from build123d import *

# Parameters (mm, degrees)
SKETCH1_R           = 3.175
BOSS_EXTRUDE1_DEPTH = 6.35


with BuildPart() as part:
    # Sketch1 → Boss-Extrude1 (new body)
    with BuildSketch(Plane.XY):
        Polygon((38.1, 12.7), (114.3, 12.7), (114.3, 17.050166685), (139.7, 17.050166685), (139.7, 12.7), (152.4, 12.7), (152.4, 0), (0, 0), (0, 12.7), (12.7, 12.7), (12.7, 17.050166685), (38.1, 17.050166685), align=None)
        with Locations((50.8, 6.35)):
            Circle(SKETCH1_R, mode=Mode.SUBTRACT)
        with Locations((76.2, 6.35)):
            Circle(SKETCH1_R, mode=Mode.SUBTRACT)
        with Locations((101.6, 6.35)):
            Circle(SKETCH1_R, mode=Mode.SUBTRACT)
    extrude(amount=BOSS_EXTRUDE1_DEPTH)


solid = part.part
Input: part model. Units: mm. Frame: model coordinates. A direction names the side the tool comes from. Coordinates: 2 decimals unless noted, no trailing zeros. Loops run counter-clockwise (first coordinate to the right, second up) from the corner with the lowest first, then second, coordinate; pieces in that order, holes last. Notation, with made-up numbers: (12, -30.75) -> (71, -30.75) arc R25 ccw to (71, -8.75) -> close; hole circle Ø3 at (-24.75, 29). An arc over 180 degrees is marked (long way). Write each question's results on one line, items separated by ' | '. Start each with the question number.
Q1. Pull-direction query (Y, two-part tool) for faces 6 (the flat face through (127, 17.05, 3)), 7 (the cylindrical face through (98.43, 6.49, 3.13)), 8 (the cylindrical face through (53.83, 7.3, 3.13)), 9 (the flat face through (77, 11, 6.35)); classes: released by +Y, released by -Y, zero draft, split by the parting line, or undercut.
Q2. Section B-B, the plane x = 50.8. Return the cut outline in (y, z) (3 decimals), plus the area to 3 significant figures.
Q3. Ray query, line 1 (X direction, y = 6.25, z = 3.5); line 2 (X direction, y = 9, z = 4); line 3 (Y direction, x = 76.2, z = 3) (3 decimals). Return the intervals inside material, ascending. Write a range as from..to.
Q4. Section C-C, the plane z = 1. Return the cut outline in (x, y) (3 decimals).
Q5. Reachability of faces 1 (the flat face through (6, 12.7, 3)), 2 (the flat face through (25, 17.05, 3)), 3 (the flat face through (146, 12.7, 3)), 4 (the flat face through (114.3, 15, 3)), 5 (the flat face through (77, 11, 0)) from +Z, -Z, +X, -X, +Y, -Y: full face, straight path, thin tool, end or side. Return the list, or none.
Q6. Pin query (flat end, axial travel): pin 1 (2 mm diameter, centred on y = 16, z = 3, fed in from +X); pin 2 (3 mm diameter, centred on x = 85.5, z = 3.5, fed in from +Y); pin 3 (1 mm diameter, centred on x = 98, y = 15, fed in from +Z). Return the tip coordinate at first contact, or that it passes through.
Q7. Section A-A, the plane y = 6.35. Return the cut outline in (x, z) (3 decimals).
Found:
1) face 6: released by +Y | face 7: undercut | face 8: undercut | face 9: zero draft
2) outline: (0, 0) -> (3.175, 0) -> (3.175, 6.35) -> (0, 6.35) -> close; (9.525, 0) -> (12.7, 0) -> (12.7, 6.35) -> (9.525, 6.35) -> close | area: 40.3 mm2
3) line 1: 0..47.63, 53.97..73.03, 79.37..98.43, 104.77..152.4 | line 2: 0..49.05, 52.55..74.45, 77.95..99.85, 103.35..152.4 | line 3: 0..3.175, 9.525..12.7
4) outline: (0, 0) -> (152.4, 0) -> (152.4, 12.7) -> (139.7, 12.7) -> (139.7, 17.05) -> (114.3, 17.05) -> (114.3, 12.7) -> (38.1, 12.7) -> (38.1, 17.05) -> (12.7, 17.05) -> (12.7, 12.7) -> (0, 12.7) -> close; hole circle Ø6.35 at (50.8, 6.35); hole circle Ø6.35 at (76.2, 6.35); hole circle Ø6.35 at (101.6, 6.35)
5) face 1: +Z, -Z, -X, +Y | face 2: +Z, -Z, +X, -X, +Y | face 3: +Z, -Z, +X, +Y | face 4: +Z, -Z, +Y | face 5: -Z, +X, -X, +Y, -Y
6) pin 1: x = 139.7 | pin 2: y = 12.7 | pin 3: through
7) outline: (0, 0) -> (47.625, 0) -> (47.625, 6.35) -> (0, 6.35) -> close; (53.975, 0) -> (73.025, 0) -> (73.025, 6.35) -> (53.975, 6.35) -> close; (79.375, 0) -> (98.425, 0) -> (98.425, 6.35) -> (79.375, 6.35) -> close; (104.775, 0) -> (152.4, 0) -> (152.4, 6.35) -> (104.775, 6.35) -> close
